Study the drawing (mm; zero at the part's minimum x, y, z) and answer. A direction names the side the tool comes from. Coordinates: 2 decimals unless noted, no trailing zeros. Loops run counter-clockwise (first coordinate to the right, second up) from the corner with the lowest first, then second, coordinate; pieces in that order, holes last. Notation, with made-up numbers: (40.25, -23.75) -> (62.25, -23.75) arc R9 ccw to (62.25, -14.75) -> close; hole circle Ø1 at (61, 3.5). An arc over 180 degrees is marked (long way). Answer in a Markdown table with one row per item.
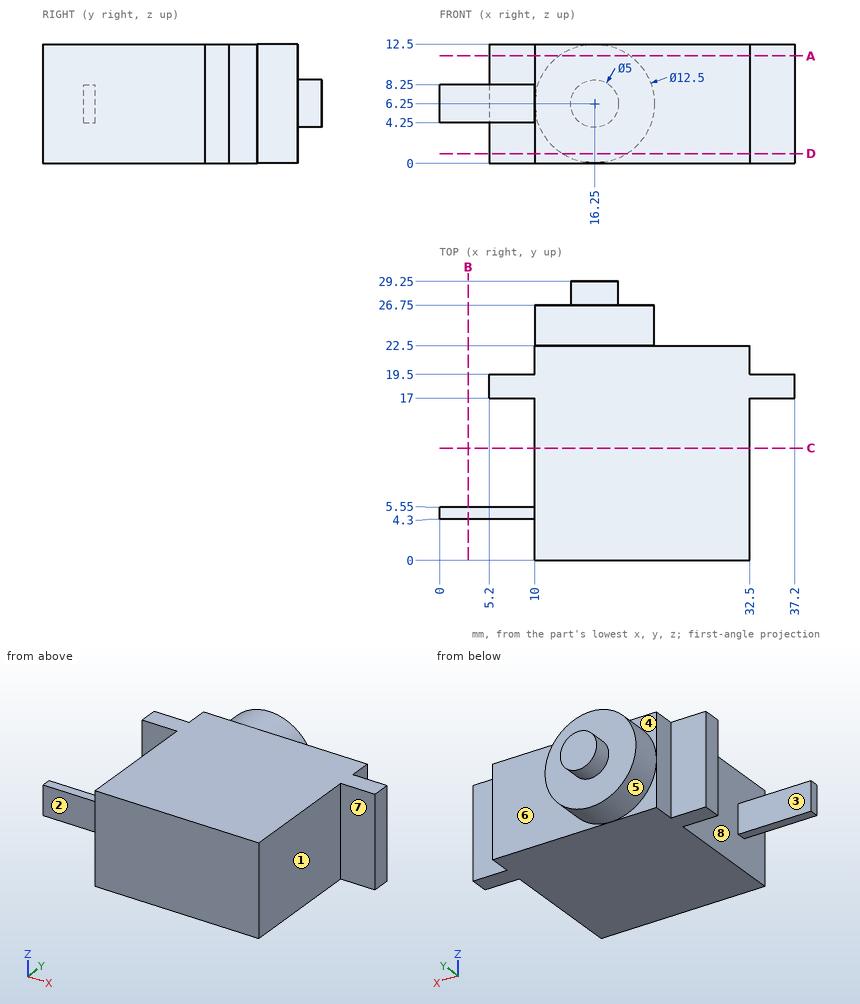
1. Find the intervals of material crossed by probe 1 along Y at (x, z) = (9.5, 4.75); probe 2 along Y at (x, z) = (34.5, 3.25); probe 3 along Y at (x, z) = (14.5, 10), in increasing order.
A:
| item | result |
|---|---|
| probe 1 | y = 4.3 to 5.55, 17 to 19.5 |
| probe 2 | y = 17 to 19.5 |
| probe 3 | y = 0 to 26.75 |
2. A cutting plane is placed at B-B on x = 3. Give the vertices of the cut face in (y, z).
A:
| item | result |
|---|---|
| outline | (4.3, 4.25) -> (5.55, 4.25) -> (5.55, 8.25) -> (4.3, 8.25) -> close |
3. A cutting plane is placed at A-A on z = 11.25. Give the vertices of the cut face in (x, y), and give its area (3 significant figures).
A:
| item | result |
|---|---|
| outline | (5.2, 17) -> (10, 17) -> (10, 0) -> (32.5, 0) -> (32.5, 17) -> (37.2, 17) -> (37.2, 19.5) -> (32.5, 19.5) -> (32.5, 22.5) -> (20, 22.5) -> (20, 26.75) -> (12.5, 26.75) -> (12.5, 22.5) -> (10, 22.5) -> (10, 19.5) -> (5.2, 19.5) -> close |
| area | 562 mm2 |
4. A cutting plane is placed at C-C on y = 11.75. Give the vertices of the cut face in (x, z), and give its area (3 significant figures).
A:
| item | result |
|---|---|
| outline | (10, 0) -> (32.5, 0) -> (32.5, 12.5) -> (10, 12.5) -> close |
| area | 281 mm2 |
5. The mould has two halves that part along Y. Classify the marked faces 6, 7 and 8: pulls with the +Y half, pulls with the -Y half, needs draft (parallel to the pull), parting line crosses it, or undercut.
A:
| item | result |
|---|---|
| face 6 | pulls with the +Y half |
| face 7 | pulls with the -Y half |
| face 8 | undercut |
6. A tool of negligible diameter and unlimited length cuts with its end or side. For the marked faces 1, 2, 3, 4 and 5, from which of +Z, -Z, +X, -X, +Y, -Y can it reach the whole face along a straight path? Write none if from no direction.
A:
| item | result |
|---|---|
| face 1 | +Z, -Z, +X, -Y |
| face 2 | +Z, -Z, -X, -Y |
| face 3 | +Z, -Z, -X |
| face 4 | +Z, -X, +Y |
| face 5 | +Y |
7. A cutting plane is placed at D-D on z = 1. Give the vertices of the cut face in (x, y).
A:
| item | result |
|---|---|
| outline | (5.2, 17) -> (10, 17) -> (10, 0) -> (32.5, 0) -> (32.5, 17) -> (37.2, 17) -> (37.2, 19.5) -> (32.5, 19.5) -> (32.5, 22.5) -> (19.64, 22.5) -> (19.64, 26.75) -> (12.86, 26.75) -> (12.86, 22.5) -> (10, 22.5) -> (10, 19.5) -> (5.2, 19.5) -> close |
8. Given pin 1 Ø1.4 at (x, z) = (35, 4) entering from -Y; pin 2 Ø2 at (y, z) = (17, 1.5) entering from -X; pin 3 Ø3.5 at (y, z) = (21, 9.5) entering from +X; pin 4 Ø3.5 at (y, z) = (21.5, 3.5) entering from -X, each flat-ended and moving along its own axis, determine where each tip first touches the part or whether it passes through.
A:
| item | result |
|---|---|
| pin 1 | stops at y = 17 |
| pin 2 | stops at x = 5.2 |
| pin 3 | stops at x = 37.2 |
| pin 4 | stops at x = 10 |
